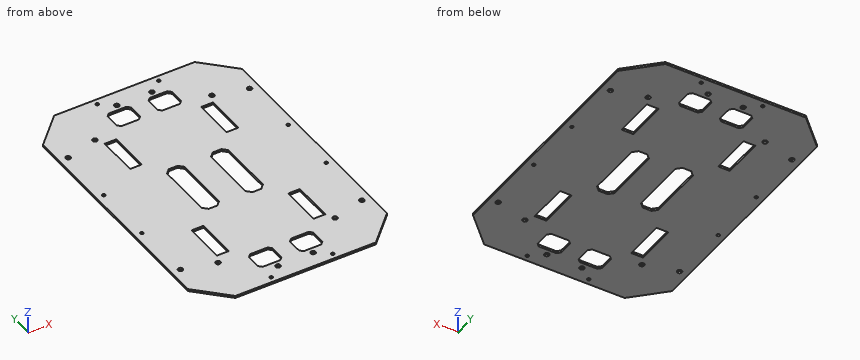
```python
from build123d import *

# Parameters (mm, degrees)
SKETCH_1_R            = 1.65
SKETCH_1_W            = 8
SKETCH_1_H            = 28
EXTRUDE_401_DEPTH     = 1.5
SKETCH_3_R            = 1.1
CUT_EXTRUDE_482_DEPTH = 1.5


with BuildPart() as part:
    # 草图1 → Extrude 401 (new body)
    with BuildSketch(Plane.XY):
        Polygon((68, 80), (48, 100), (-48, 100), (-68, 80), (-68, -80), (-48, -100), (48, -100), (68, -80), align=None)
        with Locations((-62, -62)):
            Circle(SKETCH_1_R, mode=Mode.SUBTRACT)
        with Locations((-40, -68)):
            Circle(SKETCH_1_R, mode=Mode.SUBTRACT)
        with Locations((-12, -89)):
            Circle(SKETCH_1_R, mode=Mode.SUBTRACT)
        with Locations((-62, 62)):
            Circle(SKETCH_1_R, mode=Mode.SUBTRACT)
        with Locations((-40, 68)):
            Circle(SKETCH_1_R, mode=Mode.SUBTRACT)
        with Locations((-12, 89)):
            Circle(SKETCH_1_R, mode=Mode.SUBTRACT)
        with Locations((62, -62)):
            Circle(SKETCH_1_R, mode=Mode.SUBTRACT)
        with Locations((40, -68)):
            Circle(SKETCH_1_R, mode=Mode.SUBTRACT)
        with Locations((12, -89)):
            Circle(SKETCH_1_R, mode=Mode.SUBTRACT)
        with Locations((62, 62)):
            Circle(SKETCH_1_R, mode=Mode.SUBTRACT)
        with Locations((40, 68)):
            Circle(SKETCH_1_R, mode=Mode.SUBTRACT)
        with Locations((12, 89)):
            Circle(SKETCH_1_R, mode=Mode.SUBTRACT)
        with Locations((-33, -48)):
            Rectangle(SKETCH_1_W, SKETCH_1_H, mode=Mode.SUBTRACT)
        Polygon((-20, -85), (-8, -85), (-6, -83), (-6, -73), (-8, -71), (-20, -71), (-22, -73), (-22, -83), align=None, mode=Mode.SUBTRACT)
        with Locations((-33, 48)):
            Rectangle(SKETCH_1_W, SKETCH_1_H, mode=Mode.SUBTRACT)
        Polygon((-20, 71), (-8, 71), (-6, 73), (-6, 83), (-8, 85), (-20, 85), (-22, 83), (-22, 73), align=None, mode=Mode.SUBTRACT)
        with Locations((33, -48)):
            Rectangle(SKETCH_1_W, SKETCH_1_H, mode=Mode.SUBTRACT)
        Polygon((8, -85), (20, -85), (22, -83), (22, -73), (20, -71), (8, -71), (6, -73), (6, -83), align=None, mode=Mode.SUBTRACT)
        with Locations((33, 48)):
            Rectangle(SKETCH_1_W, SKETCH_1_H, mode=Mode.SUBTRACT)
        Polygon((8, 71), (20, 71), (22, 73), (22, 83), (20, 85), (8, 85), (6, 83), (6, 73), align=None, mode=Mode.SUBTRACT)
        Polygon((-18, -22), (-12, -22), (-9, -19), (-9, 19), (-12, 22), (-18, 22), (-21, 19), (-21, -19), align=None, mode=Mode.SUBTRACT)
        Polygon((12, -22), (18, -22), (21, -19), (21, 19), (18, 22), (12, 22), (9, 19), (9, -19), align=None, mode=Mode.SUBTRACT)
    extrude(amount=EXTRUDE_401_DEPTH)

    # 草图3 → Cut-Extrude 482 (cut)
    with BuildSketch(Plane.XY):
        with Locations((-63, -21)):
            Circle(SKETCH_3_R)
        with Locations((-21, -96)):
            Circle(SKETCH_3_R)
        with Locations((-63, 21)):
            Circle(SKETCH_3_R)
        with Locations((-21, 96)):
            Circle(SKETCH_3_R)
        with Locations((63, -21)):
            Circle(SKETCH_3_R)
        with Locations((21, -96)):
            Circle(SKETCH_3_R)
        with Locations((63, 21)):
            Circle(SKETCH_3_R)
        with Locations((21, 96)):
            Circle(SKETCH_3_R)
    extrude(amount=CUT_EXTRUDE_482_DEPTH, mode=Mode.SUBTRACT)


solid = part.part
```
CAD build for the part. Positions are in the model's coordinates, mm. Round coordinates to 2 decimals unless told otherwise and drop trailing zeros. Order: outer loops, then holes, each group sorted by start corner. A loop starts at its lowest first (then second) coordinate and runs counter-clockwise, first axis right, second up. Notation, with made-up numbers: (-19.75, 8) -> (3.25, 8) arc R25 cw to (3.25, 29) -> close; hole circle Ø4 at (61.25, -23). An arc over 180 degrees is marked (long way). Write item = value, one per line.
(1) Cut at C-C (z = 1). State how many separate pieces and enclosed holes the cut face has, plus the area to 3 significant figures.
Answers follow:
separate_pieces = 1
enclosed_holes = 30
area = 23,500 mm²
(2) Flat gauge pin, fed straight in: P1, Ø3, axis at x = 62, y = -62, coming from the -Z side. Where does the tip first touch, or does it go through?
Answers follow:
P1 = through
(3) Cut at B-B (y = -77.5). Write the cut outline in (x, z), plus the area to 3 significant figures.
Answers follow:
outline = (-68, 0) -> (-22, 0) -> (-22, 1.5) -> (-68, 1.5) -> close; (-6, 0) -> (6, 0) -> (6, 1.5) -> (-6, 1.5) -> close; (22, 0) -> (68, 0) -> (68, 1.5) -> (22, 1.5) -> close
area = 156 mm²
(4) Cut at A-A (y = 14.5). Write the cut outline in (x, z), plus the area to 3 significant figures.
Answers follow:
outline = (-68, 0) -> (-21, 0) -> (-21, 1.5) -> (-68, 1.5) -> close; (-9, 0) -> (9, 0) -> (9, 1.5) -> (-9, 1.5) -> close; (21, 0) -> (68, 0) -> (68, 1.5) -> (21, 1.5) -> close
area = 168 mm²
(5) Drill centre lines: L1, parallel to Y at x = -14, z = 0.95; L2, parallel to Y at x = 30, z = 1.1; L3, parallel to Y at x = -8.5, z = 1. Where is each one in solid material? Low to high.
Answers follow:
L1 = -100 to -85, -71 to -22, 22 to 71, 85 to 100
L2 = -100 to -62, -34 to 34, 62 to 100
L3 = -100 to -85, -71 to 71, 85 to 100
